CAD build for the part. Positions are in the model's coordinates, mm. A direction names the side the tool comes from. Coordinates: 2 decimals unless noted, no trailing zeros. Loops run counter-clockwise (first coordinate to the right, second up) from the corner with the lowest first, then second, coordinate; pieces in that order, holes last. Notation, with made-up numbers: (-27.5, -35) -> (-19.5, -35) arc R24 ccw to (-19.5, -23) -> close; hole circle Ø11 at (49.25, 76). An arc over 180 degrees is marked (long way). Write each question's results on one line, items separated by ' | '.
from build123d import *

# Parameters (mm, degrees)
F1_DEPTH = 152.4
F3_DEPTH = 50.801
F5_DEPTH = 25.4


with BuildPart() as f1:
    # F0 (on Right) → F1 (new body)
    with BuildSketch(Plane.YZ):
        with BuildLine():
            Line((0, 3.175), (0, 0))
            Line((0, 0), (50.8, 0))
            Line((50.8, 0), (50.8, 50.8))
            Line((50.8, 50.8), (47.625, 50.8))
            Line((47.625, 50.8), (47.625, 6.35))
            ThreePointArc((47.625, 6.35), (46.695064, 4.104936), (44.45, 3.175))
            Line((44.45, 3.175), (0, 3.175))
        make_face()
    extrude(amount=F1_DEPTH)

    # F2 (on face) → F3 (cut, through all)
    with BuildSketch(Plane(origin=(0, 50.8, 0), x_dir=(-1, 0, 0), z_dir=(0, 1, 0))):
        Polygon((0, 50.8), (-57.15, 50.8), (-19.05, 3.175), (-19.05, 0), (0, 0), align=None)
        Polygon((-133.35, 3.175), (-95.25, 50.8), (-152.4, 50.8), (-152.4, 0), (-133.35, 0), align=None)
    extrude(amount=-F3_DEPTH, mode=Mode.SUBTRACT)

    # F4 (on face) → F5 (cut)
    with BuildSketch(Plane.XY.offset(3.175)):
        with BuildLine():
            ThreePointArc((43.1419, 22.225), (38.1, 27.2669), (33.0581, 22.225))
            Line((33.0581, 22.225), (43.1419, 22.225))
        make_face()
        with BuildLine():
            Line((43.1419, 22.225), (33.0581, 22.225))
            ThreePointArc((33.0581, 22.225), (38.1, 17.1831), (43.1419, 22.225))
        make_face()
        with BuildLine():
            Line((109.2581, 22.225), (119.3419, 22.225))
            ThreePointArc((119.3419, 22.225), (114.3, 27.2669), (109.2581, 22.225))
        make_face()
        with BuildLine():
            ThreePointArc((109.2581, 22.225), (114.3, 17.1831), (119.3419, 22.225))
            Line((119.3419, 22.225), (109.2581, 22.225))
        make_face()
    extrude(amount=-F5_DEPTH, mode=Mode.SUBTRACT)


solid = f1.part
1) Two-plate mould, pull along X, no slides. Class faces 3 (the flat face through (76, 49, 50.8)), 4 (the flat face through (19.05, 26, 2)), 5 (the flat face through (114.57, 49.08, 26.65)), 6 (the cylindrical face through (33.443, 24.156, 1.61)): pulls with the +X half, pulls with the -X half, needs draft (parallel to the pull), parting line crosses it, or undercut.
Outcome:
face 3: needs draft | face 4: pulls with the -X half | face 5: pulls with the +X half | face 6: undercut
2) Slice it at A-A (x = 75). Write the cut outline in (y, z) (3 decimals), then the cut area to 3 significant figures.
Outcome:
outline: (0, 0) -> (50.8, 0) -> (50.8, 50.8) -> (47.625, 50.8) -> (47.625, 6.35) arc R3.175 cw to (44.45, 3.175) -> (0, 3.175) -> close | area: 315 mm^2
3) Pin check, flat tips, straight feed: pin 1 (6 mm diameter, centred on x = 117.5, y = 34, fed in from +Z) (3 decimals); pin 2 (13.5 mm diameter, centred on x = 83, z = 33, fed in from -Y) (3 decimals); pin 3 (6 mm diameter, centred on y = 45, z = 15.5, fed in from +X). Stop position of each tip, or through.
Outcome:
pin 1: stops at z = 3.175 | pin 2: stops at y = 47.625 | pin 3: stops at x = 124.65
4) Which spindle directions (+Z, -Z, +X, -X, +Y, -Y) get a long thin tool onto all of the face, cutting with end or side? Do faces 1 (the flat face through (133.35, 26, 2)), 2 (the flat face through (75, 47.625, 24)). Say none if no direction does.
Outcome:
face 1: +Z, -Z, +X, +Y, -Y | face 2: +Z, +X, -X, -Y
5) Drill centre lines: L1, parallel to Y at x = 38.1, z = 0.8; L2, parallel to Z at x = 98.5, y = 43.5 (3 decimals); L3, parallel to Y at x = 55, z = 20 (3 decimals). Where is each one in solid material? Low to high. Write a range as from..to.
Outcome:
L1: y = 0..17.18, 27.27..50.8 | L2: z = 0..3.175 | L3: y = 47.625..50.8
6) Slice it at B-B (y = 20.5). Write the cut outline in (x, z) (3 decimals), then the cut area to 3 significant figures.
Outcome:
outline: (19.05, 0) -> (33.362, 0) -> (33.362, 3.175) -> (19.05, 3.175) -> close; (42.838, 0) -> (109.562, 0) -> (109.562, 3.175) -> (42.838, 3.175) -> close; (119.038, 0) -> (133.35, 0) -> (133.35, 3.175) -> (119.038, 3.175) -> close | area: 303 mm^2
7) Slice it at D-D (z = 16). Write the cut outline in (x, y) (3 decimals).
Outcome:
outline: (29.31, 47.625) -> (123.09, 47.625) -> (123.09, 50.8) -> (29.31, 50.8) -> close
